The drawing under review shows one solid part. Ordinate dimensions are in mm from its lowest x, y, z. A direction names the side the tool comes from. Coordinates: 2 decimals unless noted, no trailing zeros. Loops run counter-clockwise (first coordinate to the right, second up) from the corner with the lowest first, then second, coordinate; pieces in that order, holes last. Notation, with made-up numbers: M 46,70 L 58,70 A27 cw 58,87 Z; hole C 12.25,-18 d11. An arc over 180 degrees is marked long. Return JSON: item names as keys, results as strings.
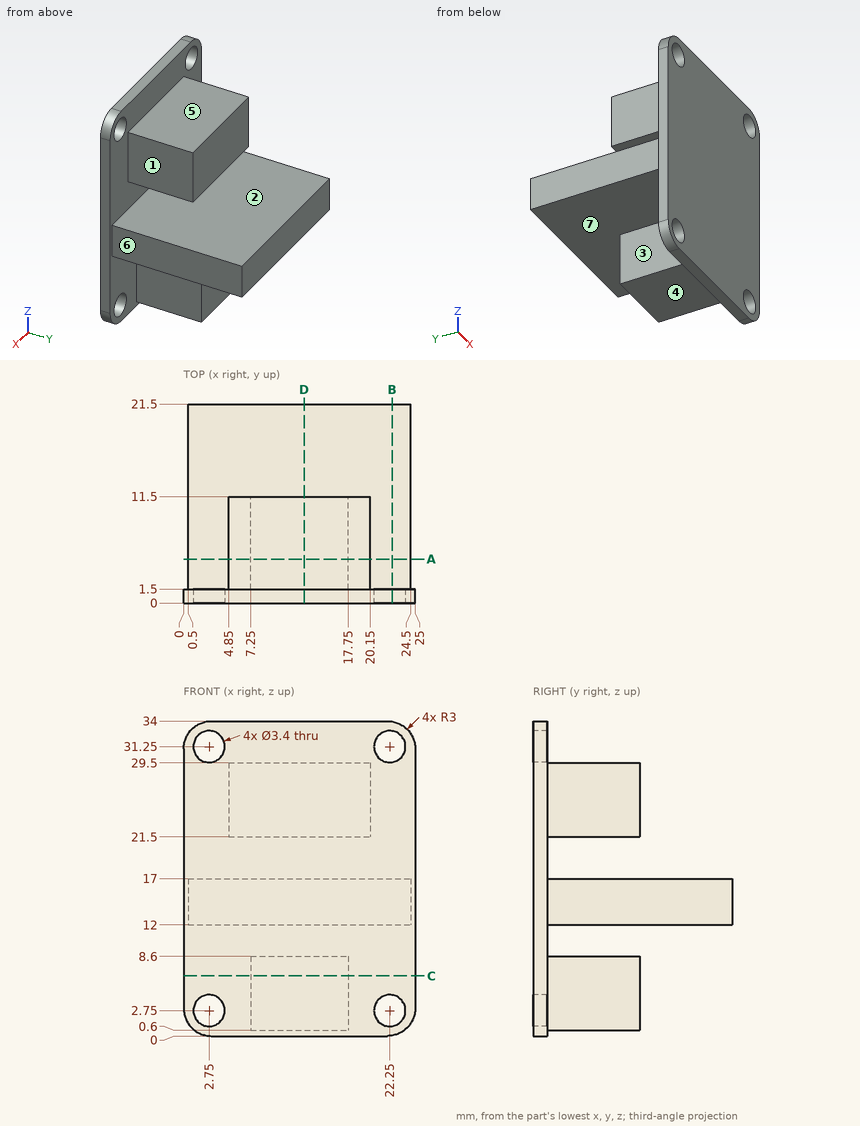
1. Insertion check: pin 1 Ø4 at (y, z) = (12, 15) entering from -X; pin 2 Ø5 at (x, y) = (14.5, 8) entering from -Z; pin 3 Ø4 at (y, z) = (5.5, 27.5) entering from +X. Each pin has a flat end and moves straight along its axis. Give the tip position at first contact, or say it passes through.
Check values:
{"pin 1": "x = 0.5", "pin 2": "z = 0.6", "pin 3": "x = 20.15"}
2. Add section B-B on x = 22.5. Give the boundary of the cut face in (y, z), plus the area to 3 significant figures.
Check values:
{"outline": "M 0,0.04 L 1.5,0.04 L 1.5,1.07 L 0,1.07 Z; M 0,4.43 L 1.5,4.43 L 1.5,12 L 21.5,12 L 21.5,17 L 1.5,17 L 1.5,29.57 L 0,29.57 Z; M 0,32.93 L 1.5,32.93 L 1.5,33.96 L 0,33.96 Z", "area": "141 mm²"}
3. Add section D-D on x = 13. Give the boundary of the cut face in (y, z), plus the area to 3 significant figures.
Check values:
{"outline": "M 0,0 L 1.5,0 L 1.5,0.6 L 11.5,0.6 L 11.5,8.6 L 1.5,8.6 L 1.5,12 L 21.5,12 L 21.5,17 L 1.5,17 L 1.5,21.5 L 11.5,21.5 L 11.5,29.5 L 1.5,29.5 L 1.5,34 L 0,34 Z", "area": "311 mm²"}
4. To check wall thickness, follow line 1 (Z direction, x = 14.5, y = 10.25); line 2 (X direction, y = 0.9, z = 31.25); line 3 (Z direction, x = 18, y = 5.25). State the ranges of each line that lie inside material, in increasing order.
Check values:
{"line 1": "0.6 to 8.6, 12 to 17, 21.5 to 29.5", "line 2": "0.01 to 1.05, 4.45 to 20.55, 23.95 to 24.99", "line 3": "12 to 17, 21.5 to 29.5"}
5. The part is to be moulded in two halves that separate along Z. For the marked faces 4, 5, 6 and 7, say which applies: released by +Z, released by -Z, zero draft, split by the parting line, or undercut.
Check values:
{"face 4": "released by -Z", "face 5": "released by +Z", "face 6": "zero draft", "face 7": "undercut"}
6. Machinability: for the marked faces 1, 2 and 3, which of the approach directions +Z, -Z, +X, -X, +Y, -Y give a long, thin tool a straight path to every point of the face, cutting with its end or side? Answer none if there is none.
Check values:
{"face 1": "+Z, +X, +Y", "face 2": "+X, -X, +Y", "face 3": "-Z, -X, +Y"}
7. Add section C-C on z = 6.5. Give the boundary of the cut face in (x, y).
Check values:
{"outline": "M 0,0 L 25,0 L 25,1.5 L 17.75,1.5 L 17.75,11.5 L 7.25,11.5 L 7.25,1.5 L 0,1.5 Z"}
8. Add section A-A on y = 4.75. Give the boundary of the cut face in (x, z).
Check values:
{"outline": "M 0.5,12 L 24.5,12 L 24.5,17 L 0.5,17 Z; M 4.85,21.5 L 20.15,21.5 L 20.15,29.5 L 4.85,29.5 Z; M 7.25,0.6 L 17.75,0.6 L 17.75,8.6 L 7.25,8.6 Z"}
